For this review, take the finished solid that the model builds, in its own axes (mm). Face numbers are marked on the shaded views. A direction names the side the tool comes from. Coordinates: 2 decimals unless noted, no trailing zeros. Order: outer loops, then holes, each group sorted by start corner. A loop starts at its lowest first (then second) coordinate and runs counter-clockwise, first axis right, second up. Notation, with made-up numbers: (29, -9.75) - (85, -9.75) arc R25 cw to (85, 11.25) - close; hole circle Ø3 at (65, -25.75). An arc over 180 degrees is marked (long way). One line per item, written item: value. Start each with the question number.
(1) Consider section B-B on x = -30. Write out the cut boundary in (y, z).
(2) For the marked faces 4, 5, 6, 7 and 8, list the 3-axis set-ups (+Z, -Z, +X, -X, +Y, -Y) from which the entire face can be reached by the end or side of a thin tool; tool diameter is ignored.
(3) To check wall thickness, follow line 1 along Y through (x, z) = (0, 14); line 2 along X through (y, z) = (-60, 13); line 3 along X through (y, z) = (42, 17.5). State the ranges of each line that lie inside material, in increasing order.
(4) Consider section A-A on x = 0. Write out the cut boundary in (y, z), then the cut area to 3 significant figures.
(5) Clearance check with flat-ended pins moving along their axes: pin 1 (3 mm diameter, centred on x = -31.5, z = 9, fed in from +Y); pin 2 (8 mm diameter, centred on y = -112, z = 12.5, fed in from -X); pin 3 (2 mm diameter, centred on x = -55, z = 14, fed in from -Y). State where each tip first meets the part, or that it passes through.
(6) Mouldability with a two-part tool opening along X and no side actions: class the marked faces 1, 2 and 3 as released by +X, released by -X, zero draft, split by the parting line, or undercut.
(7) Consider section D-D on z = 15.5. Count the separate pieces of the cut face and the enclosed holes in it, then the cut area to 3 significant figures.
```python
from build123d import *

# Parameters (mm, degrees)
F0_R     = 140
F1_DEPTH = 20
F3_DEPTH = 10
F4_R     = 1.25
F5_DEPTH = 10.001
F6_R     = 4
F7_DEPTH = 20.001


with BuildPart() as f1:
    # F0 (on Top) → F1 (new body)
    with BuildSketch(Plane.XY):
        Circle(F0_R)
    extrude(amount=F1_DEPTH)

    # F2 (on face) → F3 (cut)
    with BuildSketch(Plane.XY.offset(20)):
        with BuildLine():
            Line((-36, 135.2922762023), (-36, 100))
            ThreePointArc((-36, 100), (0, 64), (36, 100))
            Line((36, 100), (36, 135.2922762023))
            ThreePointArc((36, 135.2922762023), (0, 140), (-36, 135.2922762023))
        make_face()
        with BuildLine():
            Line((70.2102418221, 121.1219300675), (45.2548339959, 96.1665222414))
            ThreePointArc((45.2548339959, 96.1665222414), (44.6678642757, 45.8556615799), (94.9513362933, 44.0950719587))
            Line((94.9513362933, 44.0950719587), (121.9787816378, 68.7108203281))
            ThreePointArc((121.9787816378, 68.7108203281), (99.6036459707, 98.382486802), (70.2102418221, 121.1219300675))
        make_face()
        with BuildLine():
            Line((-70.2376639838, -121.1060302301), (-46.3264134966, -97.1947797428))
            ThreePointArc((-46.3264134966, -97.1947797428), (-44.7351788606, -45.7853207833), (-96.1665222414, -45.2548339959))
            Line((-96.1665222414, -45.2548339959), (-121.1219300675, -70.2102418221))
            ThreePointArc((-121.1219300675, -70.2102418221), (-99.0061557596, -98.9837417039), (-70.2376639838, -121.1060302301))
        make_face()
        with BuildLine():
            Line((135.2922762023, 36), (100, 36))
            ThreePointArc((100, 36), (64, 0), (100, -36))
            Line((100, -36), (135.2922762023, -36))
            ThreePointArc((135.2922762023, -36), (140, 0), (135.2922762023, 36))
        make_face()
        with BuildLine():
            Line((-135.2922762023, -36), (-100, -36))
            ThreePointArc((-100, -36), (-64, 0), (-100, 36))
            Line((-100, 36), (-135.2922762023, 36))
            ThreePointArc((-135.2922762023, 36), (-140, 0), (-135.2922762023, -36))
        make_face()
        with BuildLine():
            Line((36, -135.2922762023), (36, -100))
            ThreePointArc((36, -100), (0, -64), (-36, -100))
            Line((-36, -100), (-36, -135.2922762023))
            ThreePointArc((-36, -135.2922762023), (0, -140), (36, -135.2922762023))
        make_face()
        with BuildLine():
            Line((121.1219300675, -70.2102418221), (96.1665222414, -45.2548339959))
            ThreePointArc((96.1665222414, -45.2548339959), (45.2548339959, -45.2548339959), (45.2548339959, -96.1665222414))
            Line((45.2548339959, -96.1665222414), (70.2102418221, -121.1219300675))
            ThreePointArc((70.2102418221, -121.1219300675), (98.9949493661, -98.9949493661), (121.1219300675, -70.2102418221))
        make_face()
        with BuildLine():
            Line((-121.1219300675, 70.2102418221), (-96.1665222414, 45.2548339959))
            ThreePointArc((-96.1665222414, 45.2548339959), (-45.2548339959, 45.2548339959), (-45.2548339959, 96.1665222414))
            Line((-45.2548339959, 96.1665222414), (-70.2102418221, 121.1219300675))
            ThreePointArc((-70.2102418221, 121.1219300675), (-98.9949493661, 98.9949493661), (-121.1219300675, 70.2102418221))
        make_face()
    extrude(amount=-F3_DEPTH, mode=Mode.SUBTRACT)

    # F4 (on face) → F5 (cut, through all)
    with BuildSketch(Plane.XY.offset(10)):
        with Locations((-18, -77.9487010796)):
            Circle(F4_R)
        with Locations((18, -77.9487010796)):
            Circle(F4_R)
    extrude(amount=-F5_DEPTH, mode=Mode.SUBTRACT)

    # F6 (on face) → F7 (cut, through all)
    with BuildSketch(Plane.XY.offset(20)):
        with Locations((30, 0)):
            Circle(F6_R)
        with Locations((0, -30)):
            Circle(F6_R)
        with Locations((-30, 0)):
            Circle(F6_R)
        with Locations((0, 30)):
            Circle(F6_R)
    extrude(amount=-F7_DEPTH, mode=Mode.SUBTRACT)


solid = f1.part
```
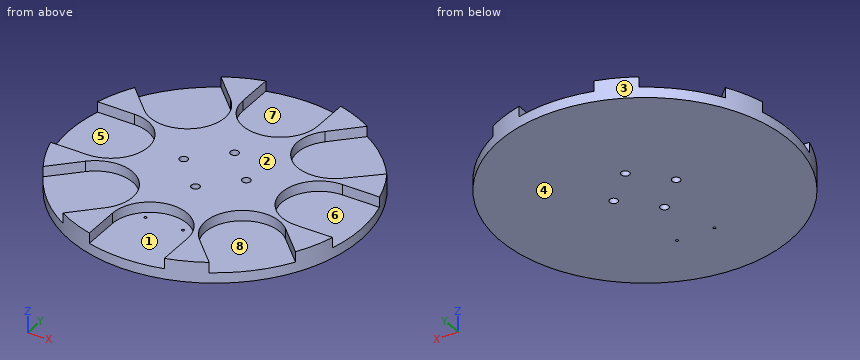
Geometry check:
1. outline: (-136.75, 0) - (-4, 0) - (-4, 20) - (-80.1, 20) - (-80.1, 10) - (-136.75, 10) - close; (4, 0) - (136.75, 0) - (136.75, 10) - (80.1, 10) - (80.1, 20) - (4, 20) - close
2. face 4: -Z, +X, -X, +Y, -Y
2. face 5: +Z, -X
2. face 6: +Z, +X
2. face 7: +Z, +Y
2. face 8: +Z
3. line 1: y = -64 to -34, -26 to 26, 34 to 64
3. line 2: x = -126.49 to -110.91, -36.34 to 36.34, 110.91 to 126.49
3. line 3: x = -133.55 to -92.43, -48.99 to 48.99, 92.43 to 133.55
4. outline: (-140, 0) - (-34, 0) - (-34, 20) - (-64, 20) - (-64, 10) - (-140, 10) - close; (-26, 0) - (26, 0) - (26, 20) - (-26, 20) - close; (34, 0) - (140, 0) - (140, 10) - (64, 10) - (64, 20) - (34, 20) - close
4. area: 3,760 mm^2
5. pin 1: stops at y = 136.75
5. pin 2: stops at x = -88.01
5. pin 3: stops at y = -129.17
6. face 1: undercut
6. face 2: zero draft
6. face 3: split by the parting line
7. separate pieces: 1
7. enclosed holes: 4
7. area: 22,900 mm^2
